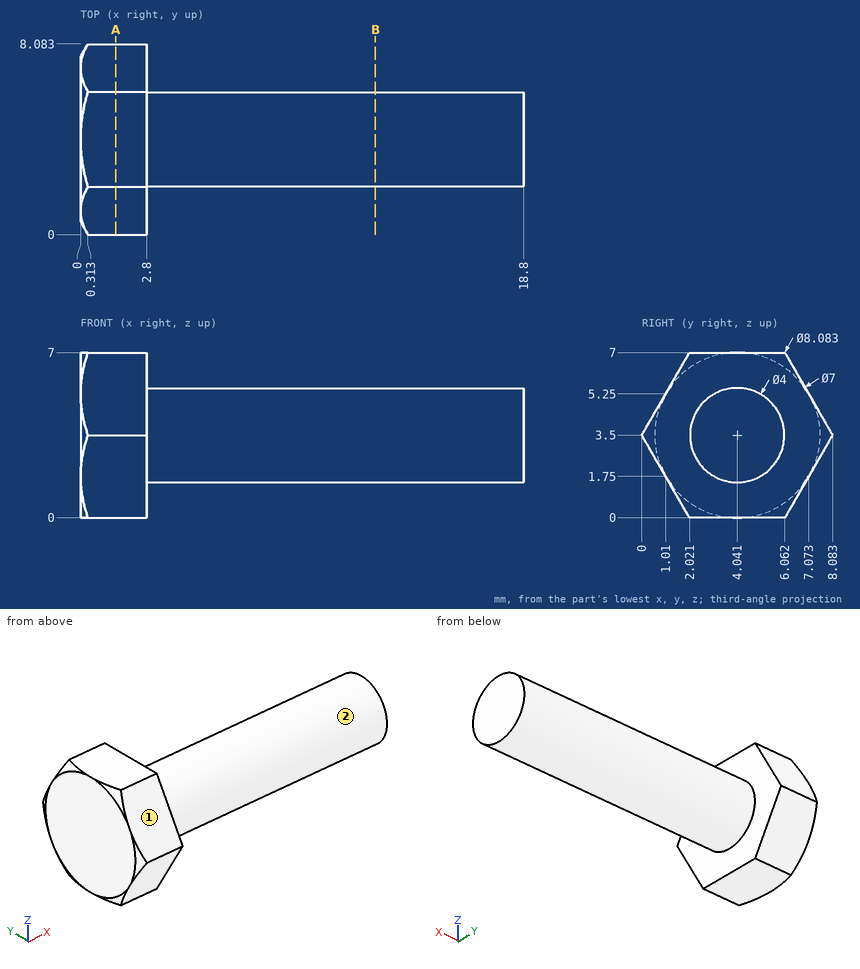
Geometry check sheet. Reference: drawing and pictorial views, mm from the part's lowest x, y, z. A direction names the side the tool comes from. Coordinates: 2 decimals unless noted, no trailing zeros. Write each loop counter-clockwise with the first axis right and the second up, starting at its lowest first coordinate (ties: lowest second). Pieces come first, ordered by that corner, then holes. Notation, with made-up numbers: M 14.5,80 L 25.5,80 A34 ccw 25.5,115 Z; hole C 53,-9.75 d8. An arc over 180 degrees is marked long. Write item = value, one per line. Start each with the question number.
1. Go/stop test with flat-tipped pins: pin 1 (2 mm diameter, centred on x = 15, z = 6, fed in from -Y); pin 2 (3 mm diameter, centred on x = 2, y = 6.5, fed in from +Z); pin 3 (2 mm diameter, centred on x = 9, y = 2.5, fed in from -Z) (1 decimal). Record where each tip stops, or that it passes through.
2. Sectioned sample at A-A (x = 1.5). Record the cut outline in (y, z).
3. Sectioned sample at B-B (x = 12.5). Record the cut outline in (y, z).
4. Tool access check on the marked faces 1 and 2. Record the directions out of +Z, -Z, +X, -X, +Y, -Y that give a thin tool (end or side, any length) a straight path to the whole face; none if there is none.
5. Thickness scan on probe 1 along X at (y, z) = (6.75, 5); probe 2 along Z at (x, y) = (8, 5) (1 decimal); probe 3 along Y at (x, z) = (15.25, 3) (1 decimal). Record the ranges inside material, lowest first.
The answers:
q1.pin_1 = 2.72
q1.pin_2 = 7
q1.pin_3 = 1.6
q2.outline = M 0,3.5 L 2.02,0 L 6.06,0 L 8.08,3.5 L 6.06,7 L 2.02,7 Z
q3.outline = C 4.04,3.5 d4
q4.face_1 = +Z, +X, -X, -Y
q4.face_2 = +X
q5.probe_1 = 0 to 2.8
q5.probe_2 = 1.7 to 5.3
q5.probe_3 = 2.1 to 6
